```python
from build123d import *

# Parameters (mm, degrees)
F0_R     = 9.906
F1_DEPTH = 3.429


# Not quite as in the source:
# - ends of sketch curves that miss each other by under 0.0002 mm in the source are joined


with BuildPart() as f1:
    # F0 (on Front) → F1 (new body)
    with BuildSketch(Plane.XZ):
        with BuildLine():
            ThreePointArc((121.3266326526, 283.5242564606), (141.1053673826, 282.2278907762), (159.8746336835, 288.5991978658))
            Line((159.8746336835, 288.5991978658), (164.9830584, 291.548566))
            Line((164.9830584, 291.548566), (165.4761232, 293.3886436))
            Line((165.4761232, 293.3886436), (306.5495774, 255.588135))
            Line((306.5495774, 255.588135), (310.4939942, 270.308832))
            Line((310.4939942, 270.308832), (169.4205146, 308.109366))
            Line((169.4205146, 308.109366), (169.9135794, 309.9494436))
            Line((169.9135794, 309.9494436), (166.9642076, 315.0578916))
            ThreePointArc((166.9642076, 315.0578916), (153.8951945869, 329.9602399108), (136.1181216974, 338.7269230379))
            Line((136.1181216974, 338.7269230379), (33.7705954, 366.1508552))
            Line((33.7705954, 366.1508552), (-68.5769266, 338.726907))
            ThreePointArc((-68.5769266, 338.726907), (-86.3539881192, 329.9602324429), (-99.4229877342, 315.0578894835))
            Line((-99.4229877342, 315.0578894835), (-102.3723632, 309.9494436))
            Line((-102.3723632, 309.9494436), (-101.8792984, 308.109366))
            Line((-101.8792984, 308.109366), (-242.952778, 270.308832))
            Line((-242.952778, 270.308832), (-239.0083612, 255.588135))
            Line((-239.0083612, 255.588135), (-97.934907, 293.3886436))
            Line((-97.934907, 293.3886436), (-97.4418676, 291.548566))
            Line((-97.4418676, 291.548566), (-92.3334196, 288.5991942))
            ThreePointArc((-92.3334196, 288.5991942), (-73.5641511826, 282.2278907762), (-53.7854164526, 283.5242564606))
            Line((-53.7854164526, 283.5242564606), (33.7705954, 306.9848318))
            Line((33.7705954, 306.9848318), (121.3266326526, 283.5242564606))
        make_face()
        Polygon((-232.4312598, 267.2114544), (-214.0303568, 272.1419754), (-213.044278, 268.4617948), (-231.4451556, 263.5312992), align=None, mode=Mode.SUBTRACT)
        Polygon((-99.9448598, 302.7110786), (-81.5439822, 307.6415996), (-80.557878, 303.961419), (-98.9587556, 299.030898), align=None, mode=Mode.SUBTRACT)
        Polygon((280.5854688, 268.4617948), (281.571573, 272.1419754), (299.972476, 267.2114544), (298.9863718, 263.5312992), align=None, mode=Mode.SUBTRACT)
        Polygon((167.486076, 302.7110786), (166.4999718, 299.030898), (148.0990942, 303.961419), (149.0851984, 307.6415996), align=None, mode=Mode.SUBTRACT)
        Polygon((-39.8353026, 318.8173964), (-21.434425, 323.747892), (-20.4483208, 320.0677114), (-38.8491984, 315.1372158), align=None, mode=Mode.SUBTRACT)
        with Locations((33.7705954, 336.5678308)):
            Circle(F0_R, mode=Mode.SUBTRACT)
        Polygon((87.989537, 320.0677114), (88.9756158, 323.747892), (107.3765188, 318.8173964), (106.3904146, 315.1372158), align=None, mode=Mode.SUBTRACT)
    extrude(amount=F1_DEPTH)


solid = f1.part
```
Verification items for the finished model (mm, model axes). A direction names the side the tool comes from. Coordinates: 2 decimals unless noted, no trailing zeros. Write each loop counter-clockwise with the first axis right and the second up, starting at its lowest first coordinate (ties: lowest second). Pieces come first, ordered by that corner, then holes. Notation, with made-up numbers: M 89.5,64 L 96.5,64 A34 cw 96.5,96 Z; hole C 65.25,3 d5. An arc over 180 degrees is marked long. Answer as a JSON object with one key per item and string values. Group by question number.
(1) Tool access check on faces 4 (the face through (235.03, -1.69, 274.75)), 5 (the face through (-86.13, -1.69, 330.13)). Record the directions out of +Z, -Z, +X, -X, +Y, -Y that give a thin tool (end or side, any length) a straight path to the whole face; none if there is none.
(2) Cross-section at C-C, the plane x = -160. Record the cut outline in (y, z).
(3) Release check for a two-part mould opening along X. For faces 1 (the face through (32, -3.429, 315)), 2 (the face through (240.945, -1.69, 288.944)), 3 (the face through (76.936, -1.69, 295.419)) record: +X half, -X half, draft (parallel to the pull), parting line (faces both ways), or undercut.
(4) Cross-section at B-B, the plane y = -2.5. State how many separate pieces and enclosed holes the cut face has, and give its area (3 significant figures).
(5) Material ranges on line 1 (Z direction, x = 92, y = -2.5); line 2 (Z direction, x = -38, y = -1); line 3 (X direction, y = -2.7, z = 335), recorded low to high.
(6) Gauge pin test, flat ends, axial feed: pin 1 (16 mm diameter, centred on x = 33.77, z = 336.57, fed in from -Y); pin 2 (1.5 mm diameter, centred on y = -1, z = 317.5, fed in from -X). Record the tip position at first contact, or that the pin passes through.
(7) Cross-section at A-A, the plane x = 28.5. Record the cut outline in (y, z).
Reply:
{
 "1": {"face 4": "-Z, +Y, -Y", "face 5": "+Z, -X, +Y, -Y"},
 "2": {"outline": "M -3.43,276.76 L 0,276.76 L 0,292.54 L -3.43,292.54 Z"},
 "3": {"face 1": "draft", "face 2": "+X half", "face 3": "undercut"},
 "4": {"separate pieces": "1", "enclosed holes": "7", "area": "18,600 mm²"},
 "5": {"line 1": "291.38 to 318.99, 322.94 to 350.55", "line 2": "287.75 to 315.36, 319.31 to 346.92", "line 3": "-78.34 to 23.99, 43.55 to 145.88"},
 "6": {"pin 1": "through", "pin 2": "x = -98.4"},
 "7": {"outline": "M -3.43,305.57 L 0,305.57 L 0,328.18 L -3.43,328.18 Z; M -3.43,344.96 L 0,344.96 L 0,364.74 L -3.43,364.74 Z"}
}
